Here's the drawing with two shaded views (mm, measured from the low corner). I have some questions. Coordinates: 2 decimals unless noted, no trailing zeros. Loops run counter-clockwise (first coordinate to the right, second up) from the corner with the lowest first, then second, coordinate; pieces in that order, holes last.
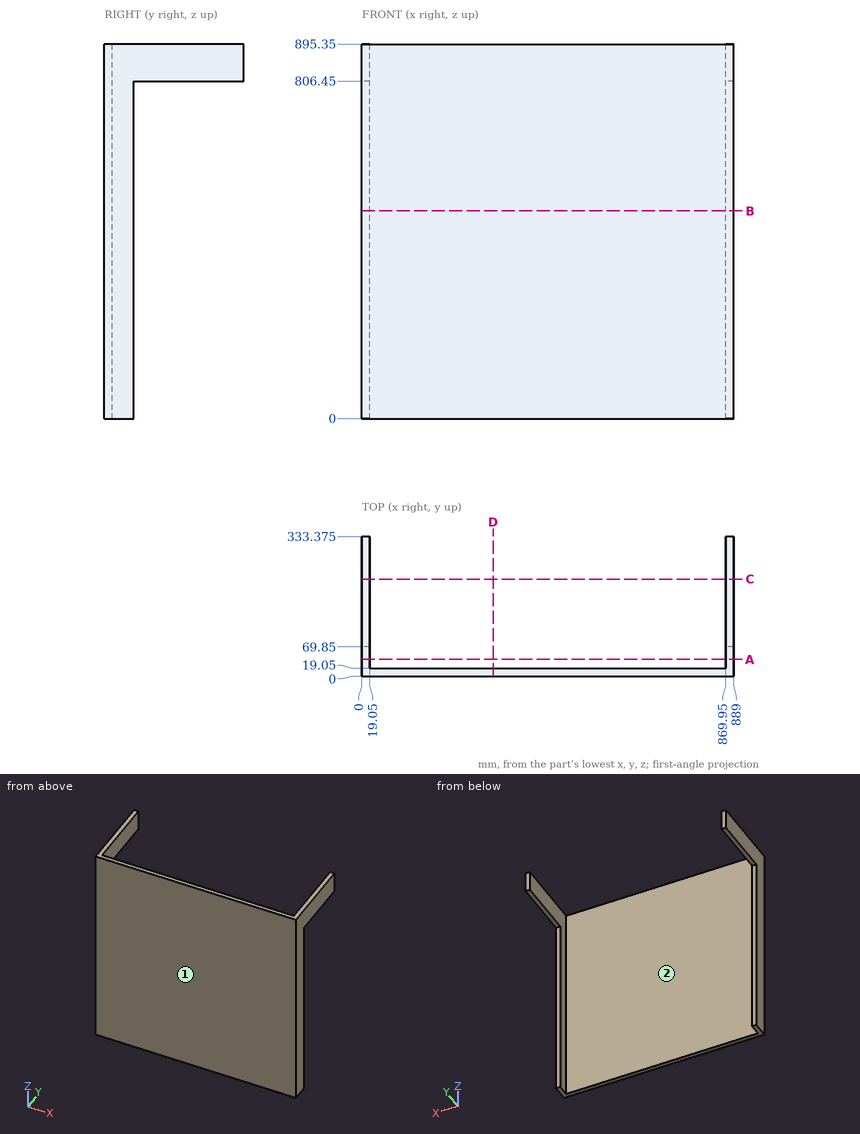
(1) I'm going to push flat-ended pins straight in: pin 1 (9.5 mm diameter, centred on x = 875.5, y = 238.5, fed in from -Z); pin 2 (21 mm diameter, centred on x = 880, z = 442, fed in from +Y). Where does each tip first touch, or does it pass through?
Check values:
pin 1: stops at z = 806.45
pin 2: stops at y = 69.85
(2) If we mould it in two halves opening along X, with no side actions, what happens to the marked faces 1 and 2? For each: released by +X, released by -X, zero draft, split by the parting line, or undercut.
Check values:
face 1: zero draft
face 2: undercut
(3) If I drill on probe 1 along X at (y, z) = (56, 528); probe 2 along Y at (x, z) = (95.5, 528), over which ranges is the centre line in solid material (lowest first)?
Check values:
probe 1: x = 0 to 19.05, 869.95 to 889
probe 2: y = 0 to 19.05
(4) I want a section at B-B on z = 496.5. Write out the boundary of the cut face in (x, y), then the cut area to 3 significant figures.
Check values:
outline: (0, 0) - (889, 0) - (889, 69.85) - (869.95, 69.85) - (869.95, 19.05) - (19.05, 19.05) - (19.05, 69.85) - (0, 69.85) - close
area: 18,900 mm2
(5) I want a section at C-C on y = 231.5. Write out the boundary of the cut face in (x, z), then the cut area to 3 significant figures.
Check values:
outline: (0, 806.45) - (19.05, 806.45) - (19.05, 895.35) - (0, 895.35) - close; (869.95, 806.45) - (889, 806.45) - (889, 895.35) - (869.95, 895.35) - close
area: 3,390 mm2
(6) I want a section at A-A on y = 39.5. Write out the boundary of the cut face in (x, z), then the cut area to 3 significant figures.
Check values:
outline: (0, 0) - (19.05, 0) - (19.05, 895.35) - (0, 895.35) - close; (869.95, 0) - (889, 0) - (889, 895.35) - (869.95, 895.35) - close
area: 34,100 mm2
(7) I want a section at D-D on x = 314. Write out the boundary of the cut face in (y, z), then the cut area to 3 significant figures.
Check values:
outline: (0, 0) - (19.05, 0) - (19.05, 895.35) - (0, 895.35) - close
area: 17,100 mm2
